The listing builds one solid part. Answer for the finished solid, in the listing's coordinates (mm). Coordinates: 2 decimals unless noted, no trailing zeros. Write each loop counter-clockwise with the first axis right and the second up, starting at its lowest first coordinate (ties: lowest second). Pieces come first, ordered by that corner, then holes.
(1) The part is cut by section B-B on y = 55.5. Determine the outline of the cut face in (x, z).
(2) The part is cut by section A-A on x = 50. Determine the outline of the cut face in (y, z).
(3) The part is cut by section C-C on z = 2.25. Give the number of separate pieces and of enclosed holes in the cut face, plus the area to 3 significant figures.
(4) The part is cut by section D-D on y = 76. Determine the outline of the cut face in (x, z).
(5) Straight lines are drawn through the part: line 1 (X direction, y = 46, z = 1); line 2 (X direction, y = 88, z = 2.25); line 3 (X direction, y = 82, z = 1.25). For each, find the intervals that lie inside material, in ascending order.
(6) Given P1, Ø5.5, axis at x = 110.5, y = 82.5, coming from the +Z side; P2, Ø6.5, axis at x = 104, y = 38.5, coming from the +Z side; P3, Ø1, axis at x = 27, y = 57, coming from the +Z side, each flat-ended and moving along its own axis, determine where each tip first touches the part or whether it passes through.
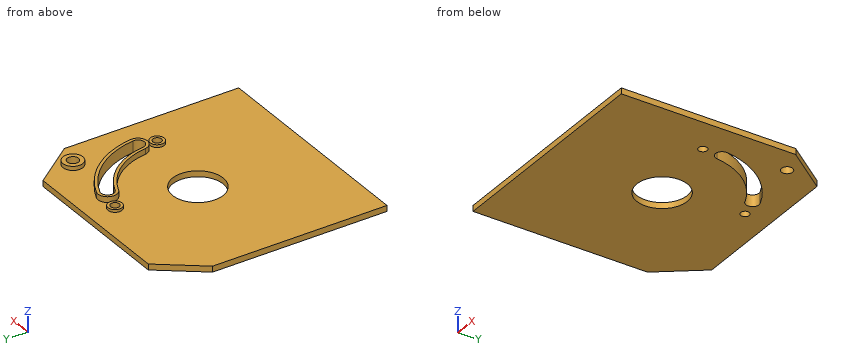
from build123d import *

# Parameters (mm, degrees)
SKETCH1_R      = 14.280154621
SKETCH1_R_2    = 3.175
SKETCH1_R_3    = 2.445943814
EXTRUDE1_DEPTH = 3.302
EXTRUDE2_DEPTH = 3.175
SKETCH3_R      = 3.969943814
SKETCH3_R_2    = 2.445943814
EXTRUDE3_DEPTH = 1.524
SKETCH4_R      = 5.604581629
SKETCH4_R_2    = 3.175
EXTRUDE4_DEPTH = 2.286


with BuildPart() as part:
    # Sketch1 → Extrude1 (new body)
    with BuildSketch(Plane.XY):
        Polygon((122.018241697, 78.932176277), (103.665120274, 103.090232189), (13.814462921, 103.090232189), (-4.538658503, 78.932176277), (-4.538658503, -19.747260734), (122.018241697, -19.747260734), align=None)
        with Locations((58.710249945, 45.283910371)):
            Circle(SKETCH1_R, mode=Mode.SUBTRACT)
        with Locations((108.031447678, 83.274598732)):
            Circle(SKETCH1_R_2, mode=Mode.SUBTRACT)
        with Locations((64.386022104, 88.408658993)):
            Circle(SKETCH1_R_3, mode=Mode.SUBTRACT)
        with Locations(Location((101.914361119, 39.6877037, 0), (0, 0, 180))):
            Circle(SKETCH1_R_3, mode=Mode.SUBTRACT)
        with BuildLine():
            ThreePointArc((105.584923307, 50.978901238), (96.144059082, 74.065464486), (76.258457488, 89.121432379))
            ThreePointArc((76.258457488, 89.121432379), (71.3691103, 86.793097674), (74.070723534, 82.099682674))
            ThreePointArc((74.070723534, 82.099682674), (90.512346787, 69.36651562), (98.311501424, 50.088712183))
            ThreePointArc((98.311501424, 50.088712183), (102.393306893, 46.897095769), (105.584923307, 50.978901238))
        make_face(mode=Mode.SUBTRACT)
    extrude(amount=EXTRUDE1_DEPTH)

    # Sketch2 → Extrude2 (add)
    with BuildSketch(Plane.XY.offset(3.302)):
        with BuildLine():
            ThreePointArc((96.672625226, 49.888999726), (89.234697097, 68.318816731), (73.552104701, 80.526896868))
            ThreePointArc((73.552104701, 80.526896868), (69.816708658, 87.358865324), (76.871357609, 90.654453557))
            ThreePointArc((76.871357609, 90.654453557), (97.452472431, 75.07236814), (107.223783381, 51.178746493))
            ThreePointArc((107.223783381, 51.178746493), (102.593085742, 45.258227686), (96.672625226, 49.888999726))
        make_face()
        with BuildLine():
            ThreePointArc((98.311501424, 50.088712183), (102.393306893, 46.897095769), (105.584923307, 50.978901238))
            ThreePointArc((105.584923307, 50.978901238), (96.144059082, 74.065464486), (76.258457488, 89.121432379))
            ThreePointArc((76.258457488, 89.121432379), (71.3691103, 86.793097674), (74.070723534, 82.099682674))
            ThreePointArc((74.070723534, 82.099682674), (90.512346787, 69.36651562), (98.311501424, 50.088712183))
        make_face(mode=Mode.SUBTRACT)
    extrude(amount=EXTRUDE2_DEPTH)

    # Sketch3 → Extrude3 (add)
    # profile 1 of 2: a face of its own
    with BuildSketch(Plane.XY.offset(3.302)):
        with Locations(Location((64.386022104, 88.408658993, 0), (0, 0, 180))):
            Circle(SKETCH3_R)
        with Locations((64.386022104, 88.408658993)):
            Circle(SKETCH3_R_2, mode=Mode.SUBTRACT)
    # profile 2 of 2: a face of its own
    with BuildSketch(Plane.XY.offset(3.302)):
        with Locations(Location((101.914361119, 39.6877037, 0), (0, 0, 180))):
            Circle(SKETCH3_R)
        with Locations(Location((101.914361119, 39.6877037, 0), (0, 0, 180))):
            Circle(SKETCH3_R_2, mode=Mode.SUBTRACT)
    extrude(amount=EXTRUDE3_DEPTH)

    # Sketch4 → Extrude4 (add)
    with BuildSketch(Plane.XY.offset(3.302)):
        with Locations(Location((108.031447678, 83.274598732, 0), (0, 0, 180))):
            Circle(SKETCH4_R)
        with Locations((108.031447678, 83.274598732)):
            Circle(SKETCH4_R_2, mode=Mode.SUBTRACT)
    extrude(amount=EXTRUDE4_DEPTH)


solid = part.part
Model answer:
1. outline: (-4.54, 0) - (48.73, 0) - (48.73, 3.3) - (-4.54, 3.3) - close; (68.69, 0) - (97.27, 0) - (97.27, 6.48) - (95.56, 6.48) - (95.56, 3.3) - (68.69, 3.3) - close; (104.81, 0) - (122.02, 0) - (122.02, 3.3) - (106.5, 3.3) - (106.5, 6.48) - (104.81, 6.48) - close
2. outline: (-19.75, 0) - (33.97, 0) - (33.97, 3.3) - (-19.75, 3.3) - close; (56.6, 0) - (103.09, 0) - (103.09, 3.3) - (56.6, 3.3) - close
3. separate pieces: 1
3. enclosed holes: 5
3. area: 14,000 mm2
4. outline: (-4.54, 0) - (84.16, 0) - (84.16, 6.48) - (81.49, 6.48) - (81.49, 3.3) - (-4.54, 3.3) - close; (94.57, 0) - (122.02, 0) - (122.02, 3.3) - (96.72, 3.3) - (96.72, 6.48) - (94.57, 6.48) - close
5. line 1: x = -4.54 to 44.45, 72.97 to 122.02
5. line 2: x = 2.35 to 61.97, 66.8 to 72.01, 78.83 to 115.13
5. line 3: x = -2.21 to 74.31, 88.4 to 105.12, 110.94 to 119.69
6. P1: stops at z = 5.59
6. P2: stops at z = 4.83
6. P3: stops at z = 3.3
